from build123d import *

# Parameters (mm, degrees)
F0_W     = 31
F0_H     = 19.05
F0_R     = 2.15265
F1_DEPTH = 9.525
F2_R     = 2.15265
F3_DEPTH = 31
F4_W     = 9.525
F4_H     = 9.525
F5_DEPTH = 3.175
F6_W     = 10.7375
F6_H     = 9.525
F7_DEPTH = 9.525
F8_R     = 4.76249


# Not quite as in the source:
# - a fillet or chamfer is up to 0.001 mm smaller than in the source, because OpenCascade refuses the exact size


with BuildPart() as f1:
    # F0 (on Top) → F1 (new body)
    with BuildSketch(Plane.XY):
        with Locations((15.5, -9.525)):
            Rectangle(F0_W, F0_H)
        with Locations((15.5, -4.7625)):
            Circle(F0_R, mode=Mode.SUBTRACT)
    extrude(amount=F1_DEPTH)

    # F2 (on face) → F3 (cut, through all)
    with BuildSketch(Plane.YZ.offset(31)):
        with Locations((-14.2875, 4.7625)):
            Circle(F2_R)
    extrude(amount=-F3_DEPTH, mode=Mode.SUBTRACT)

    # F4 (on face) → F5 (join)
    with BuildSketch(Plane(origin=(0, 0, 0), x_dir=(1, 0, 0), z_dir=(0, 0, -1))):
        with Locations((15.5, 14.2875)):
            Rectangle(F4_W, F4_H)
    extrude(amount=F5_DEPTH)

    # F6 (on face) → F7 (cut, through all)
    with BuildSketch(Plane(origin=(0, 0, 0), x_dir=(1, 0, 0), z_dir=(0, 0, -1))):
        with Locations((25.63125, 4.7625)):
            Rectangle(F6_W, F6_H)
        with Locations((5.36875, 4.7625)):
            Rectangle(F6_W, F6_H)
    extrude(amount=-F7_DEPTH, mode=Mode.SUBTRACT)

    # F8 (radius 4.7625 in the source; OpenCascade refuses exactly that, so slightly less here)
    f8_edges = [f1.edges().sort_by_distance(p)[0] for p in [
        (15.5, -19.05, 9.525),
        (25.63125, -9.525, 9.525),
        (5.36875, -9.525, 9.525),
    ]]
    fillet(f8_edges, radius=F8_R)


solid = f1.part
Read the model definition and answer for the solid it produces. Units are mm, in the model's axes. A direction names the side the tool comes from. Give positions to 0.01 mm unless a question says otherwise; leave off trailing zeros. Write each loop counter-clockwise with the first axis right and the second up, starting at its lowest first coordinate (ties: lowest second). Pieces come first, ordered by that corner, then holes. Notation, with made-up numbers: (48.5, 65) - (61.5, 65) arc R5 ccw to (61.5, 70) - close; hole circle Ø2 at (-21, -22.75). An arc over 180 degrees is marked (long way). Use CSV: the item, a comma, the result in double quotes. Start each with the question number.
(1) Determine the mould class of faces 4 (the cylindrical face through (13.35, -4.67, 4.7)), 5 (the flat face through (5, -9.525, 2)), 6 (the flat face through (15, -19.05, 2)) for opening direction Y: +Y half, -Y half, draft (parallel to the pull), parting line (faces both ways), or undercut.
(2) Find section B-B (y = -4). Give the vertices of the cut face in (x, z) (1 decimal).
(3) Find section A-A (x = 15.5). Count the separate pieces of the cut face and the enclosed holes in it, plus the area to 3 significant figures.
(4) Consider line 1 along Y through (x, z) = (15.5, 4.5); line 2 along Y through (x, z) = (22.5, 2.25) (3 decimals); line 3 along Z through (x, y) = (13.5, -14.75) (1 decimal). Determine where each line is inside the solid, lowest interval first.
(5) Given P1, Ø5, axis at x = 6.5, z = 3, coming from the +Y side (3 decimals); P2, Ø10.5, axis at x = 26.5, y = -16, coming from the -Z side; P3, Ø3.5, axis at x = 15.5, y = -4.76, coming from the +Z side; P4, Ø2, axis at x = 7, z = 6.5, coming from the +Y side, each flat-ended and moving along its own axis, determine where each tip first touches the part or whether it passes through.
(6) For faces 1 (the flat face through (26, -14, 0)), 2 (the flat face through (5, -14, 0)), 3 (the cylindrical face through (25.71, -10.96, 8.17)), determine the directions among +Z, -Z, +X, -X, +Y, -Y from which every point of the face is accessible in a straight line to the end or side of a thin tool.
Findings below:
1,face 4,"undercut"
1,face 5,"+Y half"
1,face 6,"-Y half"
2,outline,"(10.7, 0) - (13.5, 0) - (13.5, 9.5) - (10.7, 9.5) - close; (17.5, 0) - (20.3, 0) - (20.3, 9.5) - (17.5, 9.5) - close"
3,separate pieces,"2"
3,enclosed holes,"1"
3,area,"151 mm2"
4,line 1,"-19.05 to -16.42, -12.15 to -6.92, -2.61 to 0"
4,line 2,"-19.05 to -9.525"
4,line 3,"-3.2 to 2.7, 6.9 to 9.5"
5,P1,"y = -9.525"
5,P2,"z = 0"
5,P3,"through"
5,P4,"y = -9.58"
6,face 1,"-Z, +X, +Y, -Y"
6,face 2,"-Z, -X, +Y, -Y"
6,face 3,"+Z, +X, +Y"
